Drawing for the job (mm, zero at the part's lowest x, y, z). Coordinates: 2 decimals unless noted, no trailing zeros. Loops run counter-clockwise (first coordinate to the right, second up) from the corner with the lowest first, then second, coordinate; pieces in that order, holes last. Notation, with made-up numbers: (-38, 89.5) - (-9, 89.5) arc R28 cw to (-9, 107.5) - close; hole circle Ø1 at (-8.75, 6). An arc over 180 degrees is marked (long way). Put each result on its own line as item: value.
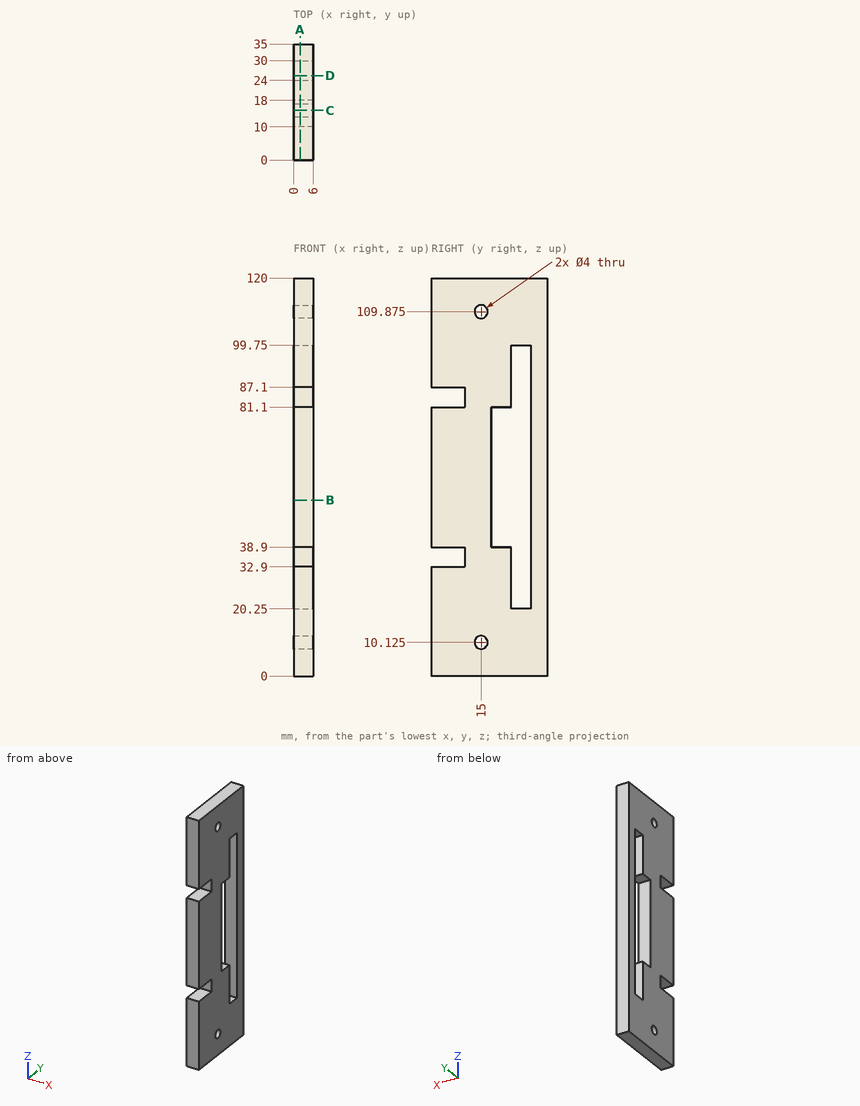
Q1. Slice it at C-C, the plane y = 15. Give the cut face in (x, z) (3 decimals).
Determined:
outline: (0, 0) - (6, 0) - (6, 8.125) - (0, 8.125) - close; (0, 12.125) - (6, 12.125) - (6, 107.875) - (0, 107.875) - close; (0, 111.875) - (6, 111.875) - (6, 120) - (0, 120) - close
Q2. Slice it at D-D, the plane y = 25.5. Give the cut face in (x, z), then the cut area to 3 significant figures.
Determined:
outline: (0, 0) - (6, 0) - (6, 20.25) - (0, 20.25) - close; (0, 99.75) - (6, 99.75) - (6, 120) - (0, 120) - close
area: 243 mm2
Q3. Slice it at B-B, the plane z = 53. Give the cut face in (x, y).
Determined:
outline: (0, 0) - (6, 0) - (6, 18) - (0, 18) - close; (0, 30) - (6, 30) - (6, 35) - (0, 35) - close
Q4. Wall check: L1, parallel to Z at x = 3.75, y = 8; L2, parallel to Y at x = 5.35, z = 44.5; L3, parallel to Y at x = 0.3, z = 83. Give the ranges that are in metal, low to high. Write a range as from..to.
Determined:
L1: 0..32.9, 38.9..81.1, 87.1..120
L2: 0..18, 30..35
L3: 10..24, 30..35
Q5. Slice it at A-A, the plane x = 2. Give the cut face in (y, z) (3 decimals), then the cut area to 3 significant figures.
Determined:
outline: (0, 0) - (35, 0) - (35, 120) - (0, 120) - (0, 87.1) - (10, 87.1) - (10, 81.1) - (0, 81.1) - (0, 38.9) - (10, 38.9) - (10, 32.9) - (0, 32.9) - close; hole circle Ø4 at (15, 10.125); hole circle Ø4 at (15, 109.875); hole (18, 38.9) - (24, 38.9) - (24, 20.25) - (30, 20.25) - (30, 99.75) - (24, 99.75) - (24, 81.1) - (18, 81.1) - close
area: 3,320 mm2
